from build123d import *

# Parameters (mm, degrees)
SKETCH1_R           = 1.55
BOSS_EXTRUDE1_DEPTH = 4.75
FILLET2_R           = 1
CUT_EXTRUDE1_DEPTH  = 3
SKETCH3_W           = 5
SKETCH3_H           = 18
BOSS_EXTRUDE2_DEPTH = 5
SKETCH8_R           = 4
SKETCH8_R_2         = 1.55
BOSS_EXTRUDE4_DEPTH = 4
SKETCH9_R           = 8
SKETCH9_R_2         = 1.55
BOSS_EXTRUDE5_DEPTH = 0.5
FILLET3_R           = 4
SKETCH7_R           = 0.95
CUT_EXTRUDE3_DEPTH  = 20.5


with BuildPart() as part:
    # Sketch1 → Boss-Extrude1 (new body)
    with BuildSketch(Plane.XY):
        with BuildLine():
            Line((-8, 0), (-8, 40))
            ThreePointArc((-8, 40), (0, 48), (8, 40))
            Line((8, 40), (8, 0))
            ThreePointArc((8, 0), (0, -8), (-8, 0))
        make_face()
        with Locations((0, 40)):
            Circle(SKETCH1_R, mode=Mode.SUBTRACT)
        Circle(SKETCH1_R, mode=Mode.SUBTRACT)
    extrude(amount=BOSS_EXTRUDE1_DEPTH)

    # Fillet2
    fillet2_edges = [part.edges().sort_by_distance(p)[0] for p in [
        (0, 48, 4.75),
        (-8, 20, 4.75),
        (0, -8, 4.75),
        (8, 20, 4.75),
    ]]
    fillet(fillet2_edges, radius=FILLET2_R)

    # Sketch2 → Cut-Extrude1 (cut)
    with BuildSketch(Plane.XY.offset(4.75)):
        Polygon((3.175426481, 40), (1.58771324, 42.75), (-1.58771324, 42.75), (-3.175426481, 40), (-1.58771324, 37.25), (1.58771324, 37.25), align=None)
        Polygon((3.175426481, 0), (1.58771324, 2.75), (-1.58771324, 2.75), (-3.175426481, 0), (-1.58771324, -2.75), (1.58771324, -2.75), align=None)
    extrude(amount=-CUT_EXTRUDE1_DEPTH, mode=Mode.SUBTRACT)

    # Sketch3 → Boss-Extrude2 (add)
    with BuildSketch(Plane(origin=(0, 0, 0), x_dir=(-1, 0, 0), z_dir=(0, 0, -1))):
        with Locations((5.5, 21)):
            Rectangle(SKETCH3_W, SKETCH3_H)
    extrude(amount=BOSS_EXTRUDE2_DEPTH)

    # Sketch8 → Boss-Extrude4 (add)
    with BuildSketch(Plane(origin=(0, 0, 0), x_dir=(-1, 0, 0), z_dir=(0, 0, -1))):
        Circle(SKETCH8_R)
        Circle(SKETCH8_R_2, mode=Mode.SUBTRACT)
    extrude(amount=BOSS_EXTRUDE4_DEPTH)

    # Sketch9 → Boss-Extrude5 (add)
    with BuildSketch(Plane(origin=(0, 0, 0), x_dir=(-1, 0, 0), z_dir=(0, 0, -1))):
        with Locations((0, 40)):
            Circle(SKETCH9_R)
        with Locations((0, 40)):
            Circle(SKETCH9_R_2, mode=Mode.SUBTRACT)
    extrude(amount=BOSS_EXTRUDE5_DEPTH)

    # Fillet3
    fillet3_edges = [part.edges().sort_by_distance(p)[0] for p in [
        (-3, 21, 0),
    ]]
    fillet(fillet3_edges, radius=FILLET3_R)

    # Mirror5: part across plane


with BuildPart() as part_1:
    add(part.part)
    add(part.part.mirror(Plane.XY.offset(-5)))

    # Sketch7 → Cut-Extrude3 (cut, through all)
    with BuildSketch(Plane(origin=(0, 0, -14.75), x_dir=(-1, 0, 0), z_dir=(0, 0, -1))):
        with Locations((-3.5, 28)):
            Circle(SKETCH7_R)
        with Locations((3.5, 28)):
            Circle(SKETCH7_R)
    extrude(amount=-CUT_EXTRUDE3_DEPTH, mode=Mode.SUBTRACT)


solid = part_1.part
Source: CAD feature listing. Evaluate the final solid. Frame: model axes, mm. A direction names the side the tool comes from. Give positions to 0.01 mm unless a question says otherwise; leave off trailing zeros. Write each loop counter-clockwise with the first axis right and the second up, starting at its lowest first coordinate (ties: lowest second). Pieces come first, ordered by that corner, then holes. Notation, with made-up numbers: (-24, 32) -> (-11, 32) arc R23 cw to (-11, 61) -> close; hole circle Ø11 at (43.5, -12.5). An arc over 180 degrees is marked (long way). Return JSON: item names as keys, results as strings. Group by question number.
1. Section B-B, the plane z = -2. Output: boundary loops of the cut face in (x, y), then the cut area to 3 significant figures.
2. Section A-A, the plane y = 6. Output: boundary loops of the cut face in (x, z), then the cut area to 3 significant figures.
3. Section D-D, the plane x = 0. Count the separate pieces of the cut face and the enclosed holes in it, then the cut area to 3 significant figures.
4. Material intervals for line 1 (X direction, y = 40, z = -0.3); line 2 (Z direction, x = -1.5, y = 2); line 3 (Z direction, x = -1, y = 32.5), sorted ascending. Write a range as from..to.
5. Section C-C, the plane y = 12.5. Output: boundary loops of the cut face in (x, z).
6. Access query for faces 1 (the face through (0, -2.75, -13)), 2 (the face through (-4.4, 28.3, -5.1)), 3 (the face through (0, 37.25, 3)), 4 (the face through (-3, 29, -5)), 5 (the face through (-2, 40, -9.5)). Directions: +Z, -Z, +X, -X, +Y, -Y. A direction counts if a zero-diameter tool reaches every point of the face in a straight line with its end or side. Return the directions, or none.
7. Pin query (flat end, axial travel): pin 1 Ø4 at (x, z) = (-4, -9) entering from +Y; pin 2 Ø1.6 at (x, y) = (-0.5, 41) entering from +Z; pin 3 Ø1.9 at (x, y) = (0, 40) entering from +Z; pin 4 Ø6 at (x, z) = (-4, -8) entering from -Y. Return the tip coordinate at first contact, or that it passes through.
8. Mould query, pull axis X, two halves, no side actions, for faces 6 (the face through (1.041, 47.932, -11.655)), 7 (the face through (-2.39, 38.64, 3.27)), 8 (the face through (7.715, 19.72, -14.449)), 9 (the face through (3.706, 27.073, 2.342)). Classes: +X half, -X half, draft (parallel to the pull), parting line (faces both ways), or undercut.
Determined:
{
 "1": {"outline": "(-8, 12) -> (-2.46, 12) -> (-2.46, 30) -> (-8, 30) -> close; circle Ø8 at (0, 0); hole circle Ø1.9 at (-3.5, 28); hole circle Ø3.1 at (0, 0)", "area": "140 mm2"},
 "2": {"outline": "(-8, -13.75) arc R1 ccw to (-7, -14.75) -> (7, -14.75) arc R1 ccw to (8, -13.75) -> (8, -10) -> (-8, -10) -> close; (-8, 0) -> (8, 0) -> (8, 3.75) arc R1 ccw to (7, 4.75) -> (-7, 4.75) arc R1 ccw to (-8, 3.75) -> close", "area": "151 mm2"},
 "3": {"separate pieces": "6", "enclosed holes": "0", "area": "500 mm2"},
 "4": {"line 1": "x = -8..-1.55, 1.55..8", "line 2": "z = -11.75..-6, -4..1.75", "line 3": "z = -14.75..-9.5, -0.5..4.75"},
 "5": {"outline": "(-8, -13.75) arc R1 ccw to (-7, -14.75) -> (7, -14.75) arc R1 ccw to (8, -13.75) -> (8, -10) -> (1, -10) arc R4 cw to (-3, -6) -> (-3, -4) arc R4 cw to (1, 0) -> (8, 0) -> (8, 3.75) arc R1 ccw to (7, 4.75) -> (-7, 4.75) arc R1 ccw to (-8, 3.75) -> close"},
 "6": {"face 1": "-Z", "face 2": "+Z, -Z", "face 3": "+Z", "face 4": "+X, +Y, -Y", "face 5": "+X, -X, +Y"},
 "7": {"pin 1": "stops at y = 47.73", "pin 2": "stops at z = 1.75", "pin 3": "passes through", "pin 4": "stops at y = -7.8"},
 "8": {"face 6": "parting line", "face 7": "undercut", "face 8": "+X half", "face 9": "undercut"}
}
